Build history of the part. All positions in model axes, mm. Round coordinates to 2 decimals unless told otherwise and drop trailing zeros. Loops run counter-clockwise (first coordinate to the right, second up) from the corner with the lowest first, then second, coordinate; pieces in that order, holes last. Notation, with made-up numbers: (-7.75, 21) - (48.25, 21) arc R11 cw to (48.25, 42) - close; hole circle Ø10 at (-14, 55.25). An arc over 180 degrees is marked (long way). Use one line per item in the form item = value. Start each with the question number.
Q1. Saw through at C-C (z = 1). Count the separate pieces of the cut face and the enclosed holes in it, then the cut area to 3 significant figures.
Q2. Mould opens along Y. For faces 1 (the face through (16.38, 95.22, 0.99)), 2 (the face through (25.97, 90, 1)), 3 (the face through (25.684, 99.582, 0.986)) say: released by +Y, released by -Y, zero draft, split by the parting line, or undercut.
Q3. Pin check, flat tip, straight feed: pin 1 (1 mm diameter, centred on x = 12, z = 1, fed in from -Y). Stop position of the tip, or through.
Q4. Drill centre lines: line 1 (Y direction, x = 16.75, z = 0.9); line 2 (Y direction, x = 6.25, z = 0.9); line 3 (X direction, y = 80, z = 1.6). Where is each one in solid material? Low to high.
Q5. Saw through at A-A (x = 16.75). Give the cut face in (y, z).
Q6. Saw through at B-B (y = 79.25). Give the cut face in (x, z).
```python
from build123d import *

# Parameters (mm, degrees)
SKETCH1_R           = 1.75
SKETCH1_R_2         = 1.7
BOSS_EXTRUDE1_DEPTH = 2


with BuildPart() as part:
    # Sketch1 → Boss-Extrude1 (new body)
    with BuildSketch(Plane.XY):
        with BuildLine():
            Line((4.131111122, 75.901391956), (25.032343796, 75.901377896))
            add(Edge.make_bspline(
                [(25.032343796, 75.901377896), (25.297692054, 75.90975298), (25.553711765, 76.028856816), (25.820691784, 76.317696861), (25.890807327, 76.431822393), (25.982618937, 76.678782523), (26.004172908, 76.809695074), (25.999986548, 76.942331771)],
                knots=[0, 0, 0, 0, 0.5, 0.5, 0.75, 0.75, 1, 1, 1, 1], degree=3))
            Line((25.999986548, 76.942331771), (25.999989945, 81.991990504))
            Line((25.999989945, 81.991990504), (25.969599942, 81.991985956))
            Line((25.969599942, 81.991985956), (25.969599942, 98.882300825))
            ThreePointArc((25.969599942, 98.882300825), (25.676706723, 99.589407606), (24.969599942, 99.882300825))
            Line((24.969599942, 99.882300825), (3.969599942, 99.882300825))
            ThreePointArc((3.969599942, 99.882300825), (3.282219087, 99.579042106), (2.999989942, 98.882762708))
            Line((2.999989942, 98.882762708), (2.999989942, 81.988548625))
            Line((2.999989942, 81.988548625), (2.999986426, 76.761900171))
            add(Edge.make_bspline(
                [(2.999986426, 76.761900171), (3.018498442, 76.630517465), (3.062890006, 76.50357159), (3.194804967, 76.27757553), (3.283868214, 76.176461233), (3.492056184, 76.01738597), (3.61249117, 75.958146472), (3.866997461, 75.89099095), (3.999692385, 75.882874863), (4.131111122, 75.901391956)],
                knots=[0, 0, 0, 0, 0.25, 0.25, 0.5, 0.5, 0.75, 0.75, 1, 1, 1, 1], degree=3))
        make_face()
        with Locations(Location((6.240524228, 78.941533895, 0), (0, 0, 180))):
            Circle(SKETCH1_R, mode=Mode.SUBTRACT)
        with Locations((16.749987873, 78.911635363)):
            Circle(SKETCH1_R_2, mode=Mode.SUBTRACT)
        with Locations((16.749999958, 96.877378149)):
            Circle(SKETCH1_R_2, mode=Mode.SUBTRACT)
        with Locations((6.240524228, 96.835747978)):
            Circle(SKETCH1_R, mode=Mode.SUBTRACT)
    extrude(amount=BOSS_EXTRUDE1_DEPTH)


solid = part.part
```
Report:
q1.separate_pieces = 1
q1.enclosed_holes = 4
q1.area = 513 mm²
q2.face_1 = undercut
q2.face_2 = zero draft
q2.face_3 = released by +Y
q3.pin_1 = 75.9
q4.line_1 = 75.9 to 77.21, 80.61 to 95.18, 98.58 to 99.88
q4.line_2 = 75.9 to 77.19, 80.69 to 95.09, 98.59 to 99.88
q4.line_3 = 3 to 4.85, 7.63 to 15.44, 18.06 to 26
q5.outline = (75.9, 0) - (77.21, 0) - (77.21, 2) - (75.9, 2) - close; (80.61, 0) - (95.18, 0) - (95.18, 2) - (80.61, 2) - close; (98.58, 0) - (99.88, 0) - (99.88, 2) - (98.58, 2) - close
q6.outline = (3, 0) - (4.52, 0) - (4.52, 2) - (3, 2) - close; (7.96, 0) - (15.08, 0) - (15.08, 2) - (7.96, 2) - close; (18.42, 0) - (26, 0) - (26, 2) - (18.42, 2) - close
